```python
from build123d import *

# Parameters (mm, degrees)
F0_W        = 3.875
F0_H        = 7.4
F0_R        = 1.17
F0_W_2      = 15.5
F1_DEPTH    = 0.4
F2_DEPTH    = 6.4
F3_W        = 3.6
F3_H        = 3.75
F4_DEPTH    = 0.5
F3_W_2      = 5.4
F5_DEPTH    = 5.5
F6_T1_DEPTH = 16.25
F7_DEPTH    = 0.5


# Not quite as in the source:
# - a fillet or chamfer that OpenCascade refuses, or shapes differently, is made with other operations: its cross-section is extruded or revolved along the edge and cut away or added


with BuildPart() as f1:
    # F0 (on Top) → F1 (new body)
    with BuildSketch(Plane.XY):
        with Locations((-9.6875, 0)):
            Rectangle(F0_W, F0_H)
        with Locations((-9.505, 0)):
            Circle(F0_R, mode=Mode.SUBTRACT)
        Rectangle(F0_W_2, F0_H)
        with Locations((9.6875, 0)):
            Rectangle(F0_W, F0_H)
        with Locations((9.505, 0)):
            Circle(F0_R, mode=Mode.SUBTRACT)
    extrude(amount=-F1_DEPTH)

    # F0 (on Top) → F2 (join)
    with BuildSketch(Plane.XY):
        Rectangle(F0_W_2, F0_H)
    extrude(amount=F2_DEPTH)

    # F3 (on face) → F4 (cut)
    with BuildSketch(Plane(origin=(0, 0, -0.4), x_dir=(1, 0, 0), z_dir=(0, 0, -1))):
        with Locations((2.7, 0)):
            Rectangle(F3_W, F3_H)
    extrude(amount=-F4_DEPTH, mode=Mode.SUBTRACT)

    # F3 (on face) → F5 (join)
    with BuildSketch(Plane(origin=(0, 0, -0.4), x_dir=(1, 0, 0), z_dir=(0, 0, -1))):
        with Locations((-1.8, 0)):
            Rectangle(F3_W_2, F3_H)
    extrude(amount=F5_DEPTH)

    # F6: fillet of radius 2.5 on 2 edges, made by hand

    # F6_s2 → F6_t1 (cut)
    with BuildSketch(Plane.XZ.offset(-8.125)):
        with BuildLine():
            add(Edge.make_bspline(
                [(-4.5, -3.4), (-4.5, -5.9), (-2, -5.9)],
                knots=[0, 0, 0, 1, 1, 1], degree=2, weights=[1, 3, 1]))
            Line((-2, -5.9), (-4.5, -5.9))
            Line((-4.5, -5.9), (-4.5, -3.4))
        make_face()
        with BuildLine():
            add(Edge.make_bspline(
                [(0.9, -3.4), (0.9, -5.9), (-1.6, -5.9)],
                knots=[0, 0, 0, 1, 1, 1], degree=2, weights=[1, 3, 1]))
            Line((-1.6, -5.9), (0.9, -5.9))
            Line((0.9, -5.9), (0.9, -3.4))
        make_face()
    extrude(amount=F6_T1_DEPTH, mode=Mode.SUBTRACT)

    # F3 (on face) → F7 (cut)
    with BuildSketch(Plane(origin=(0, 0, -0.4), x_dir=(1, 0, 0), z_dir=(0, 0, -1))):
        with Locations((2.7, 0)):
            Rectangle(F3_W, F3_H)
    extrude(amount=-F7_DEPTH, mode=Mode.SUBTRACT)


solid = f1.part
```
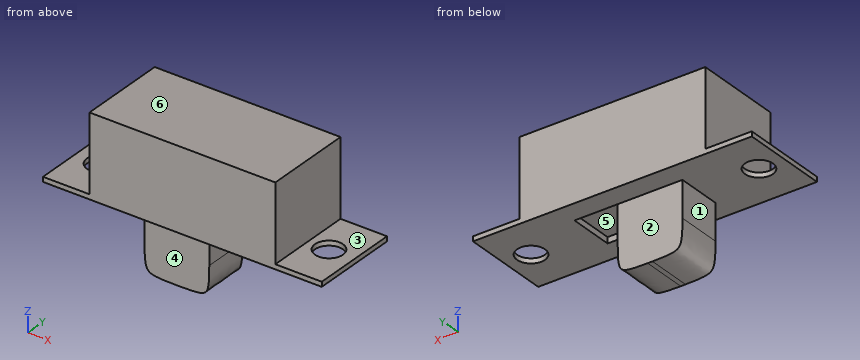
Geometry check sheet. Reference: the model listing, model coordinates, mm. Face numbers are marked on the shaded views. A direction names the side the tool comes from. Give positions to 0.01 mm unless a question says otherwise; leave off trailing zeros. Order: outer loops, then holes, each group sorted by start corner. A loop starts at its lowest first (then second) coordinate and runs counter-clockwise, first axis right, second up. Notation, with made-up numbers: (50.25, 85) -> (104.25, 85) arc R22 ccw to (104.25, 123) -> close; hole circle Ø9 at (2, 0.25). An arc over 180 degrees is marked (long way). Write each question's results on one line, items separated by ' | '. Start each with the question number.
(1) Gauge pin test, flat ends, axial feed: P1, Ø3, axis at y = -0.5, z = 3, coming from the +X side; P2, Ø2.5, axis at y = -0.5, z = -2, coming from the -X side; P3, Ø1.9, axis at x = -9.505, y = 0, coming from the -Z side; P4, Ø1.8, axis at y = 0.5, z = -2, coming from the +X side. Record the tip position at first contact, or that the pin passes through.
(2) Scan lines: line 1 (Z direction, x = 5.25, y = 1.25); line 2 (X direction, y = 1, z = -2.25); line 3 (X direction, y = -2.25, z = 3.25). Record each from-to range of solid material in increasing order.
(3) Mould release check, pull along Y, two halves, no side actions. Record for the marked faces 4, 5 and 6: pulls with the +Y half, pulls with the -Y half, needs draft (parallel to the pull), parting line crosses it, or undercut.
(4) Access from +Z, -Z, +X, -X, +Y, -Y to the whole of each face (thin tool, end or side, straight path). Record for the marked faces 1, 2 and 3.
(5) Sectioned sample at C-C (x = 3.5). Enter the section's corners in (y, z) (3 decimals), plus the area to 3 significant figures.
(6) Sectioned sample at B-B (y = 0). Give the number of separate pieces and of enclosed holes in the cut face, plus the area to 3 significant figures.
(7) Sectioned sample at D-D (z = 3). Enter the section's corners in (x, y).
(8) Sectioned sample at A-A (x = -9.25). Enter the section's corners in (y, z), plus the area to 3 significant figures.
Answer below:
1) P1: x = 7.75 | P2: x = -4.5 | P3: through | P4: x = 0.9
2) line 1: -0.4 to 6.4 | line 2: -4.5 to 0.9 | line 3: -7.75 to 7.75
3) face 4: pulls with the -Y half | face 5: undercut | face 6: needs draft
4) face 1: -Z, -X, +Y, -Y | face 2: -Z, +X, -X, +Y | face 3: +Z, +X, +Y, -Y
5) outline: (-3.7, -0.4) -> (-1.875, -0.4) -> (-1.875, 0.1) -> (1.875, 0.1) -> (1.875, -0.4) -> (3.7, -0.4) -> (3.7, 6.4) -> (-3.7, 6.4) -> close | area: 48.4 mm2
6) separate pieces: 3 | enclosed holes: 0 | area: 134 mm2
7) outline: (-7.75, -3.7) -> (7.75, -3.7) -> (7.75, 3.7) -> (-7.75, 3.7) -> close
8) outline: (-3.7, -0.4) -> (-1.14, -0.4) -> (-1.14, 0) -> (-3.7, 0) -> close; (1.14, -0.4) -> (3.7, -0.4) -> (3.7, 0) -> (1.14, 0) -> close | area: 2.05 mm2
